Here's how the part is built. I have some questions about the finished solid (model axes, mm). Give positions to 0.01 mm unless a question says otherwise; leave off trailing zeros. Write each loop counter-clockwise with the first axis right and the second up, starting at its lowest first coordinate (ties: lowest second). Pieces come first, ordered by that corner, then holes. Notation, with made-up numbers: M 28,-8.5 L 80,-8.5 A20 ccw 80,-2.5 Z; hole C -11.75,68 d6. An arc over 180 degrees is marked long. Answer as CSV lines item,"result". Start each with the question number.
Q1. Suppose I cut it at A-A (y = 0). Write out the boundary of the cut face in (x, z), then the cut area to 3 significant figures.
Q2. Thinking about a two-plate mould opening in X: for faces 1 (the flat face through (18, 26, 0.794)), 2 (the cylindrical face through (-16.169, -27.848, -0.011)), 3 (the flat face through (16.855, 39.076, 0.011)), which applies, +X half, -X half, draft (parallel to the pull), parting line (faces both ways), or undercut?
Q3. Suppose I cut it at B-B (x = 20). Write out the boundary of the cut face in (y, z), then the cut area to 3 significant figures.
Q4. If I drill on line 1 along X through (y, z) = (31, 0.7); line 2 along Y through (x, z) = (17, 0.3); line 3 along Y through (x, z) = (3, -0.05), over which ranges is the centre line in solid material (lowest first)?
Q5. Suppose I cut it at D-D (z = 0.4). Count the separate pieces of the cut face and the enclosed holes in it, then the cut area to 3 significant figures.
Q6. Suppose I cut it at C-C (y = 44). Write out the boundary of the cut face in (x, z).
```python
from build123d import *

# Parameters (mm, degrees)
SKETCH1_R                = 39.5
BOSS_EXTRUDE1_DEPTH      = 0.79375
BOSS_EXTRUDE2_DEPTH      = 1.5875
SKETCH2_R                = 28.75
CUT_EXTRUDE1_DEPTH       = 64.739863165
M3_CLEARANCE_HOLE1_D     = 3.6
CIRPATTERN1_COUNT        = 6
M3_CLEARANCE_HOLE2_D     = 3.6
M3_CLEARANCE_HOLE2_DEPTH = 10
M3_CLEARANCE_HOLE2_TIP   = 1.081549114


with BuildPart() as part:
    # Sketch1 → Boss-Extrude1 (new, symmetric)
    with BuildSketch(Plane.XY):
        Circle(SKETCH1_R)
    extrude(amount=BOSS_EXTRUDE1_DEPTH, both=True)

    # Sketch3 → Boss-Extrude2 (add, through all)
    with BuildSketch(Plane.XY.offset(0.79375)):
        Polygon((-28.01836343, 27.842796388), (-6, 50), (6, 50), (28.01836343, 27.842796388), align=None)
    extrude(amount=-BOSS_EXTRUDE2_DEPTH)

    # Sketch2 → Cut-Extrude1 (cut, through all)
    with BuildSketch(Plane.XY.offset(0.79375)):
        Circle(SKETCH2_R)
    extrude(amount=-CUT_EXTRUDE1_DEPTH, mode=Mode.SUBTRACT)

    # M3 Clearance Hole1 (through all)
    with Locations(Plane.XY.offset(0.79375)):
        with Locations((17, -29.444863729)):
            m3_clearance_hole1 = Hole(M3_CLEARANCE_HOLE1_D / 2)

    # CirPattern1: M3 Clearance Hole1 ×6 about axis
    cirpattern1_axis = Axis((0, 0, 0), (0, 0, 1))
    for i in range(1, CIRPATTERN1_COUNT):
        add(m3_clearance_hole1.rotate(cirpattern1_axis, i * 360 / CIRPATTERN1_COUNT), mode=Mode.SUBTRACT)

    # M3 Clearance Hole2
    with Locations(Plane.XY.offset(0.79375)):
        with Locations((3, 44), (-3, 44)):
            Hole(M3_CLEARANCE_HOLE2_D / 2, depth=M3_CLEARANCE_HOLE2_DEPTH)
            with Locations((0, 0, -(M3_CLEARANCE_HOLE2_DEPTH + M3_CLEARANCE_HOLE2_TIP / 2))):  # 118° drill point
                Cone(0, M3_CLEARANCE_HOLE2_D / 2, M3_CLEARANCE_HOLE2_TIP, mode=Mode.SUBTRACT)


solid = part.part
```
Resolved:
1,outline,"M -39.5,-0.79 L -35.8,-0.79 L -35.8,0.79 L -39.5,0.79 Z; M -32.2,-0.79 L -28.75,-0.79 L -28.75,0.79 L -32.2,0.79 Z; M 28.75,-0.79 L 32.2,-0.79 L 32.2,0.79 L 28.75,0.79 Z; M 35.8,-0.79 L 39.5,-0.79 L 39.5,0.79 L 35.8,0.79 Z"
1,area,"22.7 mm^2"
2,face 1,"draft"
2,face 2,"undercut"
2,face 3,"+X half"
3,outline,"M -34.06,-0.79 L -20.65,-0.79 L -20.65,0.79 L -34.06,0.79 Z; M 20.65,-0.79 L 35.91,-0.79 L 35.91,0.79 L 20.65,0.79 Z"
3,area,"45.5 mm^2"
4,line 1,"-24.88 to -17.91, -16.09 to 16.09, 17.91 to 24.88"
4,line 2,"-35.65 to -31.24, -27.64 to -23.19, 23.19 to 27.64, 31.24 to 38.93"
4,line 3,"-39.39 to -28.59, 28.59 to 42.2, 45.8 to 50"
5,separate pieces,"1"
5,enclosed holes,"9"
5,area,"2,530 mm^2"
6,outline,"M -11.96,-0.79 L -4.8,-0.79 L -4.8,0.79 L -11.96,0.79 Z; M -1.2,-0.79 L 1.2,-0.79 L 1.2,0.79 L -1.2,0.79 Z; M 4.8,-0.79 L 11.96,-0.79 L 11.96,0.79 L 4.8,0.79 Z"
